```python
from build123d import *

# Parameters (mm, degrees)
F0_R          = 14.2875
F0_R_2        = 12.7
F2_DEPTH      = 50.8
F3_R          = 26.9875
F3_R_2        = 14.2875
F4_DEPTH      = 63.5
F4_DEPTH_BACK = 12.7
F5_SIZE       = 7.62
F7_START      = -26.67
F7_DEPTH      = 6.35
F8_R          = 1.27


with BuildPart() as f2:
    # F0 (on Top) → F2 (new body)
    with BuildSketch(Plane.XY):
        Circle(F0_R)
        Circle(F0_R_2, mode=Mode.SUBTRACT)
    extrude(amount=F2_DEPTH)

    # F3 (on face) → F4 (join, two sides)
    with BuildSketch(Plane.XY) as f4_sk:
        Circle(F3_R)
        Circle(F3_R_2, mode=Mode.SUBTRACT)
    extrude(amount=F4_DEPTH)
    extrude(f4_sk.sketch, amount=-F4_DEPTH_BACK)

    # F5
    f5_edges = [f2.edges().sort_by_distance(p)[0] for p in [
        (-26.9875, 0, 63.5),
        (-26.9875, 0, -12.7),
    ]]
    chamfer(f5_edges, length=F5_SIZE)

    # F6 (on Front) → F7 (join)
    with BuildSketch(Plane.XZ.offset(F7_START)):
        with BuildLine():
            ThreePointArc((0, 9.1674418672), (8.5704498555, 12.717438433), (12.1204464213, 21.2878882885))
            ThreePointArc((12.1204464213, 21.2878882885), (7.8117209816, 30.5551552404), (-2.0510178584, 33.233538007))
            ThreePointArc((-2.0510178584, 33.233538007), (-12.0766681836, 20.2586618626), (0, 9.1674418672))
        make_face()
        with BuildLine():
            ThreePointArc((0, 9.1674418672), (-12.0766681836, 20.2586618626), (-2.0510178584, 33.233538007))
            Line((-2.0510178584, 33.233538007), (-48.4348551439, 25.2696280601))
            ThreePointArc((-48.4348551439, 25.2696280601), (-41.8358763876, 23.4775709789), (-38.9529867456, 17.2770116073))
            ThreePointArc((-38.9529867456, 17.2770116073), (-41.32822473, 11.5426798516), (-47.0625564857, 9.1674418672))
            Line((-47.0625564857, 9.1674418672), (0, 9.1674418672))
        make_face()
        with BuildLine():
            ThreePointArc((-38.9529867456, 17.2770116073), (-41.8358763876, 23.4775709789), (-48.4348551439, 25.2696280601))
            ThreePointArc((-48.4348551439, 25.2696280601), (-55.142835005, 16.5883749689), (-47.0625564857, 9.1674418672))
            ThreePointArc((-47.0625564857, 9.1674418672), (-41.32822473, 11.5426798516), (-38.9529867456, 17.2770116073))
        make_face()
    extrude(amount=-F7_DEPTH)

    # F8
    f8_edges = [f2.edges().sort_by_distance(p)[0] for p in [
        (12.076668, 33.02, 22.317115),
        (-25.242937, 33.02, 29.251583),
        (-55.142835, 33.02, 16.588375),
        (-23.531278, 33.02, 9.167442),
    ]]
    fillet(f8_edges, radius=F8_R)


solid = f2.part
```
CAD build for the part. Positions are in the model's coordinates, mm. A direction names the side the tool comes from. Coordinates: 2 decimals unless noted, no trailing zeros. Order: outer loops, then holes, each group sorted by start corner. A loop starts at its lowest first (then second) coordinate and runs counter-clockwise, first axis right, second up. Notation, with made-up numbers: (-1, -13.5) - (14, -13.5) arc R22 ccw to (14, -0.5) - close; hole circle Ø11 at (78.25, 89.25). An arc over 180 degrees is marked (long way). Use a Markdown table: item, result. Add a question column.
(1) Pull direction X, two halves, no side cores. Call faces 4 (the face through (-7, -13, 63.5)), 5 (the face through (-13, -1, 50.8)), 6 (the face through (-14.274, 0.628, 57.061)), 7 (the face through (-55.155, 29.174, 16.757)): +X half, -X half, draft (parallel to the pull), parting line (faces both ways), or undercut.
(2) Which spindle directions (+Z, -Z, +X, -X, +Y, -Y) get a long thin tool onto all of the face, cutting with end or side? Do faces 1 (the face through (-14.274, 0.628, -6.261)), 2 (the face through (-24.918, 29.174, 29.307)), 3 (the face through (-2.75, -12.4, 25.04)). Say none if no direction does.
(3) Drill centre lines: line 1 along Y through (x, z) = (0, 33.5); line 2 along Y through (x, z) = (0, 55.5); line 3 along X through (y, z) = (-1, 58). Where is each one in solid material? Low to high. Write a range as [from, to].
(4) Saw through at A-A (y = 0). Give the cut face in (x, z).
(5) Flat gauge pins, fed straight in: pin 1 (3 mm diameter, centred on x = -24.5, z = 7.5, fed in from -Y); pin 2 (5 mm diameter, centred on y = -9.5, z = 3, fed in from -X); pin 3 (2 mm diameter, centred on x = -6.5, z = 31.5, fed in from -Y). Where does each tip first touch, or does it go through?
(6) Saw through at B-B (z = 42.5). Give the cut face in (x, y) (1 decimal).
(7) Saw through at C-C (x = -7). Count the separate pieces of the cut face and the enclosed holes in it, then the cut area to 3 significant figures.
Solved:
| question | item | result |
|---|---|---|
| 1 | face 4 | draft |
| 1 | face 5 | undercut |
| 1 | face 6 | undercut |
| 1 | face 7 | -X half |
| 2 | face 1 | -Z |
| 2 | face 2 | +Z, -X, +Y |
| 2 | face 3 | +Z, -Z |
| 3 | line 1 | y = [-26.99, -12.7], [12.7, 26.99] |
| 3 | line 2 | y = [-26.99, -14.29], [14.29, 26.99] |
| 3 | line 3 | x = [-24.85, -14.25], [14.25, 24.85] |
| 4 | outline | (-26.99, -5.08) - (-19.37, -12.7) - (-14.29, -12.7) - (-14.29, 0) - (-12.7, 0) - (-12.7, 50.8) - (-14.29, 50.8) - (-14.29, 63.5) - (-19.37, 63.5) - (-26.99, 55.88) - close; (12.7, 0) - (14.29, 0) - (14.29, -12.7) - (19.37, -12.7) - (26.99, -5.08) - (26.99, 55.88) - (19.37, 63.5) - (14.29, 63.5) - (14.29, 50.8) - (12.7, 50.8) - close |
| 5 | pin 1 | stops at y = -14.12 |
| 5 | pin 2 | stops at x = -26.06 |
| 5 | pin 3 | stops at y = -26.42 |
| 6 | outline | circle Ø54 at (0, 0); hole circle Ø25.4 at (0, 0) |
| 7 | separate pieces | 3 |
| 7 | enclosed holes | 0 |
| 7 | area | 2,290 mm² |
